from build123d import *

# Parameters (mm, degrees)
F1_DEPTH = 52
F3_W     = 54.390293
F3_H     = 10.69973
F4_DEPTH = 8
F5_W     = 54.836117
F5_H     = 11.145552
F6_DEPTH = 8


with BuildPart() as f1:
    # F0 (on Top) → F1 (new body)
    with BuildSketch(Plane.XY):
        Polygon((-31.876273, 43.913472), (-47.480047, 43.913472), (-47.480047, -32.767925), (-43.021828, -32.767925), (12.260112, -32.767925), (12.260112, -55.504851), (-49.263336, -55.504851), (-49.263336, -65.758757), (-43.467648, -65.758757), (22.514023, -65.758757), (22.514023, -32.767925), (22.514023, -19.839084), (-31.876273, -19.839084), align=None)
    extrude(amount=F1_DEPTH)

    # F3 (on Top) → F4 (join)
    with BuildSketch(Plane.XY):
        with Locations((-5.572776, 0.22291)):
            Rectangle(F3_W, F3_H)
    extrude(amount=-F4_DEPTH)

    # F5 (on offset) → F6 (join)
    with BuildSketch(Plane.XY.offset(52)):
        with Locations((-5.795691, 0.445822)):
            Rectangle(F5_W, F5_H)
    extrude(amount=F6_DEPTH)


solid = f1.part
Work out the finished part from the listing and answer in its coordinate system (mm). A direction names the side the tool comes from. Coordinates: 2 decimals unless noted, no trailing zeros. Order: outer loops, then holes, each group sorted by start corner. A loop starts at its lowest first (then second) coordinate and runs counter-clockwise, first axis right, second up. Notation, with made-up numbers: (63.5, 34) - (108.5, 34) arc R20 ccw to (108.5, 47) - close; hole circle Ø8 at (49, -9.5). An arc over 180 degrees is marked (long way). Put each result on its own line as item: value. Start each with the question number.
1) Find section A-A (x = -23.5). Give the vertices of the cut face in (y, z), plus the area to 3 significant figures.
2) For faces 5 (the flat face through (-6, 5.573, -4)), 6 (the flat face through (-47.48, 6, 26)), 7 (the flat face through (-6, 0, 0)), determine the directions among +Z, -Z, +X, -X, +Y, -Y from which every point of the face is accessible in a straight line to the end or side of a thin tool.
3) Flat-ended cylindrical pins translate along their axes: pin 1 (10 mm diameter, centred on x = 8.5, y = -24.5, fed in from -Z); pin 2 (2.5 mm diameter, centred on x = -9, z = -3.5, fed in from -Y); pin 3 (7 mm diameter, centred on y = -49.5, z = 34.5, fed in from -X); pin 4 (10 mm diameter, centred on x = -28.5, y = 9.5, fed in from -Z). Find the tip coordinate at first contact, or state that the pin passes through.
4) Find section C-C (x = 16.5). Give the vertices of the cut face in (y, z), plus the area to 3 significant figures.
5) Find section B-B (z = 28). Give the vertices of the cut face in (x, y).
6) Find the intervals of material crossed by line 1 (Y direction, x = -1, z = 5); line 2 (Y direction, x = -32, z = 45.5); line 3 (Y direction, x = 13, z = 9), in increasing order. Write a range as from..to.
7) Find section D-D (x = -41). Give the vertices of the cut face in (y, z), plus the area to 3 significant figures.
8) For a pull along Z with two mould halves and no side action, classify faces 1 (the flat face through (-6, -5.127, -4)), 2 (the flat face through (-6, 0, -8)), 3 (the flat face through (-6, 1, 60)), 4 (the flat face through (-31.876, 12, 26)) as released by +Z, released by -Z, zero draft, split by the parting line, or undercut.
Results list:
1. outline: (-65.76, 0) - (-55.5, 0) - (-55.5, 52) - (-65.76, 52) - close; (-32.77, 0) - (-19.84, 0) - (-19.84, 52) - (-32.77, 52) - close; (-5.13, -8) - (5.57, -8) - (5.57, 0) - (-5.13, 0) - close; (-5.13, 52) - (6.02, 52) - (6.02, 60) - (-5.13, 60) - close
1. area: 1,380 mm^2
2. face 5: -Z, +X, -X, +Y
2. face 6: +Z, -Z, -X, +Y
2. face 7: +X, +Y
3. pin 1: stops at z = 0
3. pin 2: stops at y = -5.13
3. pin 3: stops at x = 12.26
3. pin 4: stops at z = -8
4. outline: (-65.76, 0) - (-19.84, 0) - (-19.84, 52) - (-65.76, 52) - close; (-5.13, -8) - (5.57, -8) - (5.57, 0) - (-5.13, 0) - close; (-5.13, 52) - (6.02, 52) - (6.02, 60) - (-5.13, 60) - close
4. area: 2,560 mm^2
5. outline: (-49.26, -65.76) - (22.51, -65.76) - (22.51, -19.84) - (-31.88, -19.84) - (-31.88, 43.91) - (-47.48, 43.91) - (-47.48, -32.77) - (12.26, -32.77) - (12.26, -55.5) - (-49.26, -55.5) - close
6. line 1: y = -65.76..-55.5, -32.77..-19.84
6. line 2: y = -65.76..-55.5, -32.77..43.91
6. line 3: y = -65.76..-19.84
7. outline: (-65.76, 0) - (-55.5, 0) - (-55.5, 52) - (-65.76, 52) - close; (-32.77, 0) - (43.91, 0) - (43.91, 52) - (-32.77, 52) - close
7. area: 4,520 mm^2
8. face 1: zero draft
8. face 2: released by -Z
8. face 3: released by +Z
8. face 4: undercut
